Design review of the part built by this model. Coordinates are the model's own, in mm. Give positions to 0.01 mm unless a question says otherwise; leave off trailing zeros. Write each loop counter-clockwise with the first axis right and the second up, starting at its lowest first coordinate (ties: lowest second). Pieces come first, ordered by that corner, then holes. Notation, with made-up numbers: M -9.75,35.25 L 14.25,35.25 A27 ccw 14.25,55.25 Z; hole C -2,60.25 d2. An arc over 180 degrees is marked long. Write each question's results on one line, items separated by ' | '. Start each with the question number.
from build123d import *

# Parameters (mm, degrees)
SKETCH1_W           = 20
SKETCH1_H           = 22
BOSS_EXTRUDE1_DEPTH = 20
SKETCH2_W           = 8
SKETCH2_H           = 8
CUT_EXTRUDE1_DEPTH  = 16
SKETCH3_W           = 20
SKETCH3_H           = 5
BOSS_EXTRUDE2_DEPTH = 2
LPATTERN1_COUNT     = 6
LPATTERN1_PITCH     = 22
SKETCH4_W           = 20
SKETCH4_H           = 17
BOSS_EXTRUDE3_DEPTH = 2
SKETCH5_W           = 20
SKETCH5_H           = 22
BOSS_EXTRUDE4_DEPTH = 2
SKETCH6_W           = 118
SKETCH6_H           = 2
CUT_EXTRUDE2_DEPTH  = 2
SKETCH7_W           = 134
SKETCH7_H           = 20
BOSS_EXTRUDE5_DEPTH = 6


with BuildPart() as part:
    # Sketch1 → Boss-Extrude1 (new body)
    with BuildSketch(Plane.XY):
        with Locations((10, 11)):
            Rectangle(SKETCH1_W, SKETCH1_H)
    extrude(amount=BOSS_EXTRUDE1_DEPTH)

    # Sketch2 → Cut-Extrude1 (cut)
    with BuildSketch(Plane(origin=(0, 0, 0), x_dir=(-1, 0, 0), z_dir=(0, -1, 0))):
        with Locations((-10, -10)):
            Rectangle(SKETCH2_W, SKETCH2_H)
    extrude(amount=-CUT_EXTRUDE1_DEPTH, mode=Mode.SUBTRACT)

    # Sketch3 → Boss-Extrude2 (add)
    with BuildSketch(Plane(origin=(20, 0, 0), x_dir=(0, 0, -1), z_dir=(1, 0, 0))):
        with Locations((-10, 2.5)):
            Rectangle(SKETCH3_W, SKETCH3_H)
    extrude(amount=BOSS_EXTRUDE2_DEPTH)


with BuildPart() as lpattern1_1:
    # LPattern1: pattern copy
    add(part.part.moved(Location(Vector(1, 0, 0) * (1 * LPATTERN1_PITCH))))


with BuildPart() as lpattern1_2:
    # LPattern1: pattern copy
    add(part.part.moved(Location(Vector(1, 0, 0) * (2 * LPATTERN1_PITCH))))


with BuildPart() as lpattern1_3:
    # LPattern1: pattern copy
    add(part.part.moved(Location(Vector(1, 0, 0) * (3 * LPATTERN1_PITCH))))


with BuildPart() as lpattern1_4:
    # LPattern1: pattern copy
    add(part.part.moved(Location(Vector(1, 0, 0) * (4 * LPATTERN1_PITCH))))


with BuildPart() as lpattern1_5:
    # LPattern1: pattern copy
    add(part.part.moved(Location(Vector(1, 0, 0) * (5 * LPATTERN1_PITCH))))


with BuildPart() as lpattern1_1_1:
    add(lpattern1_1.part)

    # Combine1: union LPattern1_2, LPattern1_3, LPattern1_4, LPattern1_5, part
    add(lpattern1_2.part)
    add(lpattern1_3.part)
    add(lpattern1_4.part)
    add(lpattern1_5.part)
    add(part.part)

    # Sketch4 → Boss-Extrude3 (add)
    with BuildSketch(Plane(origin=(130, 0, 0), x_dir=(0, 0, -1), z_dir=(1, 0, 0))):
        with Locations((-10, 13.5)):
            Rectangle(SKETCH4_W, SKETCH4_H)
    extrude(amount=BOSS_EXTRUDE3_DEPTH)

    # Sketch5 → Boss-Extrude4 (add)
    with BuildSketch(Plane.ZY):
        with Locations((10, 11)):
            Rectangle(SKETCH5_W, SKETCH5_H)
    extrude(amount=BOSS_EXTRUDE4_DEPTH)

    # Sketch6 → Cut-Extrude2 (cut)
    with BuildSketch(Plane.XZ):
        with Locations((65, 10)):
            Rectangle(SKETCH6_W, SKETCH6_H)
    extrude(amount=-CUT_EXTRUDE2_DEPTH, mode=Mode.SUBTRACT)

    # Sketch7 → Boss-Extrude5 (add)
    with BuildSketch(Plane(origin=(0, 0, 0), x_dir=(-1, 0, 0), z_dir=(0, -1, 0))):
        with Locations((-65, -10)):
            Rectangle(SKETCH7_W, SKETCH7_H)
    extrude(amount=BOSS_EXTRUDE5_DEPTH)


solid = lpattern1_1_1.part
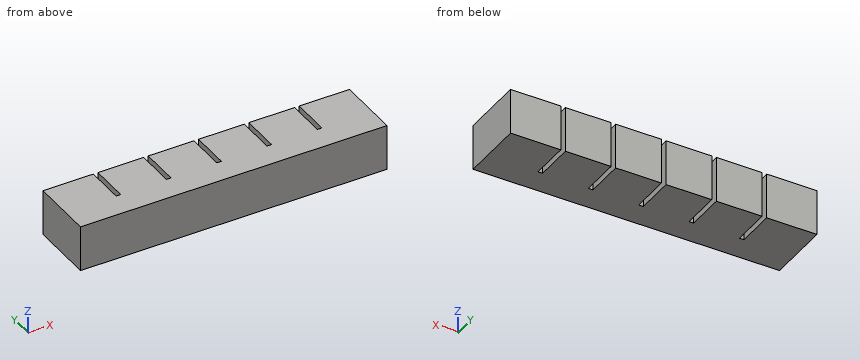
Q1. We need section A-A on y = 18. Write out the cut boundary in (x, z).
Q2. For pin 1 Ø1 at (x, z) = (21, 8.5) entering from +Y, flat-tipped, find the tip position at first contact; note if it passes through.
Q3. Wall thickness on line 1 along X through (y, z) = (8.5, 17.75); line 2 along X through (y, z) = (1.5, 10.5); line 3 along Y through (x, z) = (54, 9.5): over which ranges is each line inside the solid? List them lowest first. Write a range as from..to.
Q4. We need section B-B on x = 76. Write out the cut boundary in (y, z), and give its area (3 significant figures).
Q5. We need section C-C on z = 16. Write out the cut boundary in (x, y).
Answer sheet:
1) outline: M -2,0 L 20,0 L 20,20 L -2,20 Z; M 22,0 L 42,0 L 42,20 L 22,20 Z; M 44,0 L 64,0 L 64,20 L 44,20 Z; M 66,0 L 86,0 L 86,20 L 66,20 Z; M 88,0 L 108,0 L 108,20 L 88,20 Z; M 110,0 L 132,0 L 132,20 L 110,20 Z
2) pin 1: y = 5
3) line 1: -2..20, 22..42, 44..64, 66..86, 88..108, 110..132 | line 2: -2..6, 124..132 | line 3: -6..0, 16..22
4) outline: M -6,0 L 22,0 L 22,20 L -6,20 Z; hole M 0,6 L 16,6 L 16,14 L 0,14 Z | area: 432 mm^2
5) outline: M -2,-6 L 132,-6 L 132,22 L 110,22 L 110,5 L 108,5 L 108,22 L 88,22 L 88,5 L 86,5 L 86,22 L 66,22 L 66,5 L 64,5 L 64,22 L 44,22 L 44,5 L 42,5 L 42,22 L 22,22 L 22,5 L 20,5 L 20,22 L -2,22 Z
